```python
from build123d import *

# Parameters (mm, degrees)
BOSS_EXTRUDE1_DEPTH             = 10
F_5_1_5_1_DIAMETER_HOLE1_D      = 5.1
F_8_2_8_2_DIAMETER_HOLE1_D      = 8.2
F_5_1_5_1_DIAMETER_HOLE2_REACH  = 51.648
F_5_1_5_1_DIAMETER_HOLE2_BORE_R = 2.55
CHAMFER1_SIZE                   = 0.3
SKETCH8_R                       = 2.525
CUT_EXTRUDE1_DEPTH              = 8


with BuildPart() as part:
    # Sketch1 → Boss-Extrude1 (new body)
    with BuildSketch(Plane(origin=(28, 0, 0), x_dir=(0, -1, 0), z_dir=(-1, 0, 0))):
        with BuildLine():
            Line((-14.722431864, 3.5), (-4.330127019, -14.5))
            ThreePointArc((-4.330127019, -14.5), (0, -17), (4.330127019, -14.5))
            Line((4.330127019, -14.5), (14.722431864, 3.5))
            ThreePointArc((14.722431864, 3.5), (14.722431864, 8.5), (10.392304845, 11))
            Line((10.392304845, 11), (-10.392304845, 11))
            ThreePointArc((-10.392304845, 11), (-14.722431864, 8.5), (-14.722431864, 3.5))
        make_face()
    extrude(amount=-BOSS_EXTRUDE1_DEPTH)

    # Ø5.1 (5.1) Diameter Hole1 (through all)
    with Locations(Plane.ZY.offset(-28)):
        with Locations((-10, 0), (5, 8.660254038), (5, -8.660254038)):
            Hole(F_5_1_5_1_DIAMETER_HOLE1_D / 2)

    # Ø8.2 (8.2) Diameter Hole1 (through all)
    with Locations(Plane.ZY.offset(-28)):
        with Locations((0, 0)):
            Hole(F_8_2_8_2_DIAMETER_HOLE1_D / 2)

    # Ø5.1 (5.1) Diameter Hole2 bore → Ø5.1 (5.1) Diameter Hole2 (cut, up to next)
    with BuildSketch(Plane.XY.offset(11), mode=Mode.PRIVATE) as f_5_1_5_1_diameter_hole2_sk1:
        with Locations((33, 0)):
            Circle(F_5_1_5_1_DIAMETER_HOLE2_BORE_R)
    f_5_1_5_1_diameter_hole2_tool1 = extrude(f_5_1_5_1_diameter_hole2_sk1.sketch, amount=-F_5_1_5_1_DIAMETER_HOLE2_REACH, mode=Mode.PRIVATE) & part.part
    add(f_5_1_5_1_diameter_hole2_tool1.solids().sort_by_distance((33, 0, 11))[0], mode=Mode.SUBTRACT)

    # Chamfer1
    chamfer1_edges = [part.edges().sort_by_distance(p)[0] for p in [
        (28, -8.660254038, 7.55),
        (28, 8.660254038, 7.55),
        (28, 0, -7.45),
        (28, 0, 4.1),
        (28, 0, 11),
        (28, -14.722431864, 8.5),
        (28, -9.526279442, -5.5),
        (28, 0, -17),
        (28, 9.526279442, -5.5),
        (28, 14.722431864, 8.5),
    ]]
    chamfer(chamfer1_edges, length=CHAMFER1_SIZE)

    # Sketch8 → Cut-Extrude1 (cut)
    with BuildSketch(Plane(origin=(0, 9.526279442, -5.5), x_dir=(1, 0, 0), z_dir=(0, 0.8660254037844384, -0.5000000000000006))):
        with Locations(Location((33, -0.002304845, 0), (0, 0, 270))):
            Circle(SKETCH8_R)
    extrude(amount=-CUT_EXTRUDE1_DEPTH, mode=Mode.SUBTRACT)


solid = part.part
```
Design review of the part built by this model. Coordinates are the model's own, in mm. Coordinates: 2 decimals unless noted, no trailing zeros. Order: outer loops, then holes, each group sorted by start corner. A loop starts at its lowest first (then second) coordinate and runs counter-clockwise, first axis right, second up. Notation, with made-up numbers: (-32.5, -24) - (3.5, -24) arc R13 cw to (3.5, -14) - close; hole circle Ø10 at (-30, 54). An arc over 180 degrees is marked (long way). One line per question, with ' | ' between items.
Q1. Clearance check with flat-ended pins moving along their axes: pin 1 Ø4 at (x, z) = (35, 1.5) entering from +Y; pin 2 Ø1 at (x, z) = (33.5, -4.5) entering from +Y; pin 3 Ø4 at (x, z) = (36.5, -4) entering from -Y. State where each tip first meets the part, or that it passes through.
Answer key:
pin 1: stops at y = 14.72 | pin 2: stops at y = 3.75 | pin 3: stops at y = -11.55
Q2. Consider section C-C, the plane x = 31.25. Give the boundary of the cut face in (y, z).
Answer key:
outline: (-14.72, 3.5) - (-4.33, -14.5) arc R5 ccw to (4.33, -14.5) - (8.62, -7.07) - (2.27, -3.41) arc R4.1 cw (long way) to (-1.85, 3.66) - (-1.85, 11) - (-10.39, 11) arc R5 ccw to start; (1.85, 3.66) arc R4.1 cw to (4.09, -0.26) - (10.44, -3.92) - (14.72, 3.5) arc R5 ccw to (10.39, 11) - (1.85, 11) - close; hole circle Ø5.1 at (-8.66, 5); hole circle Ø5.1 at (0, -10); hole circle Ø5.1 at (8.66, 5)
Q3. Consider section B-B, the plane z = 5. Give the number of separate pieces and of enclosed holes in the cut face, then the cut area to 3 significant figures.
Answer key:
separate pieces: 3 | enclosed holes: 1 | area: 183 mm2
Q4. Consider section D-D, the plane z = -10. Give the boundary of the cut face in (x, y).
Answer key:
outline: (28, -6.58) - (28.3, -6.93) - (38, -6.93) - (38, -2.55) - (28.3, -2.55) - (28, -2.85) - close; (28, 2.85) - (28.3, 2.55) - (38, 2.55) - (38, 6.93) - (28.3, 6.93) - (28, 6.58) - close
Q5. Consider section A-A, the plane x = 33. Give the boundary of the cut face in (y, z).
Answer key:
outline: (-14.72, 3.5) - (-4.33, -14.5) arc R5 ccw to (4.33, -14.5) - (8.26, -7.68) - (1.54, -3.8) arc R4.1 cw to (-2.55, 3.21) - (-2.55, 11) - (-10.39, 11) arc R5 ccw to start; (2.55, 3.21) arc R4.1 cw to (4.06, 0.57) - (10.79, -3.31) - (14.72, 3.5) arc R5 ccw to (10.39, 11) - (2.55, 11) - close; hole circle Ø5.1 at (-8.66, 5); hole circle Ø5.1 at (0, -10); hole circle Ø5.1 at (8.66, 5)
Q6. To check wall thickness, follow line 1 along Y through (x, z) = (34, 5); line 2 along Z through (x, y) = (31.5, 7); line 3 along Y through (x, z) = (31.75, 5). State the ranges of each line that lie inside material, in increasing order.
Answer key:
line 1: y = -15.29 to -11.21, -6.11 to -2.35, 2.35 to 6.11, 11.21 to 15.29 | line 2: z = -9.88 to -6.38, -1.69 to 3.06, 6.94 to 11 | line 3: y = -15.29 to -11.21, -6.11 to -2.22, 2.22 to 6.11, 11.21 to 15.29
Q7. The part is to be moulded in two halves that separate along Z. For faces 1 (the cylindrical face through (33, 0, -17)), 2 (the cylindrical face through (33.22, -3.64, -1.89)), 3 (the flat face through (28, 4, -3)), say which applies: +Z half, -Z half, draft (parallel to the pull), parting line (faces both ways), or undercut.
Answer key:
face 1: -Z half | face 2: undercut | face 3: draft
